Here's how the part is built. I have some questions about the finished solid (model axes, mm). Face numbers are marked on the shaded views. Coordinates: 2 decimals unless noted, no trailing zeros. Order: outer loops, then holes, each group sorted by start corner. A loop starts at its lowest first (then second) coordinate and runs counter-clockwise, first axis right, second up. Notation, with made-up numbers: (58, 39) - (62, 39) arc R22 ccw to (62, 65) - close; hole circle Ø9 at (-19.75, -13). An arc over 180 degrees is marked (long way). Answer as CSV lines item,"result". Start each with the question number.
Item 1: I'm going to push flat-ended pins straight in: pin 1 (3 mm diameter, centred on x = 4, z = -2, fed in from -Y); pin 2 (3 mm diameter, centred on x = 1, z = 9.5, fed in from -Y). Where does each tip first touch, or does it pass through?
Item 2: Imagine slicing it at A-A on y = 0. List the corners of the cut face in (x, z) for me, and give its area (3 significant figures).
Item 3: I need wall thicknesses on line 1 (Z direction, x = 3.4, y = 0); line 2 (Y direction, x = 4.3, z = 8); line 3 (Y direction, x = 4.5, z = -6). Which ranges of each line are inside material? Lowest first, please.
Item 4: Imagine slicing it at B-B on x = 1.15. List the corners of the cut face in (y, z) for me, and give its area (3 significant figures).
Item 5: We'd pull the mould along Z, two halves only. Please class the marked faces 1, 2 and 3: pulls with the +Z half, pulls with the -Z half, needs draft (parallel to the pull), parting line crosses it, or undercut.
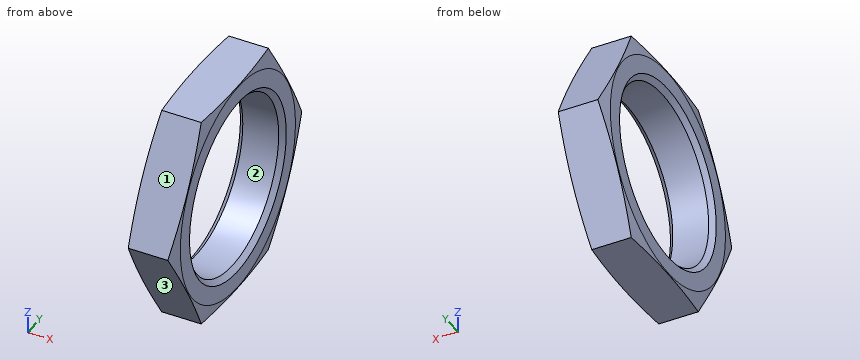
Autodesk Inventor part; units mm, degrees
ref_plane "ANBAU_XY" through (0, 0, 0) normal (1, 0, 0) x (0, 0, -1)
ref_plane "ANBAU_YZ" through (0, 0, 0) normal (0, 0, -1) x (0, 1, 0)
ref_plane "ANBAU_ZX" through (0, 0, 0) normal (0, 1, 0) x (1, 0, 0)
sketch "Skizze_1" plane through (0, 0, 0) normal (0, 0, 1) x (1, 0, 0)
  line L0 (5, 0) -> (0, 0)
  line L1 (0, 0) -> (0, 11.9)
  line L2 (0, 11.9) -> (0.864, 16.8)
  line L3 (0.864, 16.8) -> (4.136, 16.8)
  line L4 (4.136, 16.8) -> (5, 11.9)
  line L5 (5, 11.9) -> (5, 0)
  line L6 (5, 0) -> (0, 0)
revolve "Revolution1" add sketch "Skizze_1" angle 360 about axis through (5, 0, 0) along (1, 0, 0)
sketch "Skizze_3" plane through (0, 0, 0) normal (0, 0, 1) x (1, 0, 0)
  line L0 (5, 0) -> (0, 0)
  line L1 (0, 0) -> (0, 10)
  line L2 (0, 10) -> (0.5415, 9.4585)
  line L3 (0.5415, 9.4585) -> (4.4585, 9.4585)
  line L4 (4.4585, 9.4585) -> (5, 10)
  line L5 (5, 10) -> (5, 0)
  line L6 (5, 0) -> (0, 0)
revolve "Revolution2" cut sketch "Skizze_3" angle 360 about axis through (5, 0, 0) along (1, 0, 0)
thread "Thread1"
sketch "Sketch_1" plane through (0, 0, 0) normal (1, 0, 0) x (0, 1, 0)
  line L0 (24, 24) -> (-24, 24)
  line L1 (-24, 24) -> (-24, -24)
  line L2 (-24, -24) -> (24, -24)
  line L3 (24, -24) -> (24, 24)
  line L4 (-6.9282, 12) -> (-13.8564, 0)
  line L5 (-13.8564, 0) -> (-6.9282, -12)
  line L6 (-6.9282, -12) -> (6.9282, -12)
  line L7 (6.9282, -12) -> (13.8564, 0)
  line L8 (13.8564, 0) -> (6.9282, 12)
  line L9 (6.9282, 12) -> (-6.9282, 12)
extrude "Extrusion1" cut sketch "Sketch_1" along normal blind 5
ref_plane "ANBAU_XY" through (0, 0, 0) normal (1, 0, 0) x (0, 0, -1)
ref_plane "ANBAU_YZ" through (0, 0, 0) normal (0, 0, -1) x (0, 1, 0)
ref_plane "ANBAU_ZX" through (0, 0, 0) normal (0, 1, 0) x (1, 0, 0)
ref_plane "SLE_XY" through (5, 0, 0) normal (-1, 0, 0) x (0, 1, 0)
ref_plane "SLE_YZ" through (5, 0, 0) normal (0, 1, 0) x (0, 0, -1)
ref_plane "SLE_ZX" through (5, 0, 0) normal (0, 0, -1) x (-1, 0, 0)
properties part number "Flachmutter M20x1-5-24"
Responses:
1,pin 1,"stops at y = -13.57"
1,pin 2,"stops at y = -9.24"
2,outline,"(0, -11.9) - (0.02, -12) - (4.98, -12) - (5, -11.9) - (5, -10) - (4.46, -9.46) - (0.54, -9.46) - (0, -10) - close; (0, 10) - (0.54, 9.46) - (4.46, 9.46) - (5, 10) - (5, 11.9) - (4.98, 12) - (0.02, 12) - (0, 11.9) - close"
2,area,"24.8 mm^2"
3,line 1,"z = -12 to -9.46, 9.46 to 12"
3,line 2,"y = -9.24 to -5.05, 5.05 to 9.24"
3,line 3,"y = -10.39 to -7.37, 7.37 to 10.39"
4,outline,"(-13.86, 0) - (-6.93, -12) - (6.93, -12) - (13.86, 0) - (6.93, 12) - (-6.93, 12) - close; hole circle Ø18.92 at (0, 0)"
4,area,"218 mm^2"
5,face 1,"pulls with the +Z half"
5,face 2,"undercut"
5,face 3,"pulls with the -Z half"
